Verification items for the finished model (mm, model axes). A direction names the side the tool comes from. Round coordinates to 2 decimals unless told otherwise and drop trailing zeros. Loops run counter-clockwise (first coordinate to the right, second up) from the corner with the lowest first, then second, coordinate; pieces in that order, holes last. Notation, with made-up numbers: M 14,43 L 57,43 A25 ccw 57,73 Z; hole C 63,53 d10. An arc over 180 degrees is marked long. One line per item, written item: value.
from build123d import *

# Parameters (mm, degrees)
SKETCH1_R               = 8
BOSS_EXTRUDE1_DEPTH     = 16
SKETCH2_R               = 6.5
CUT_EXTRUDE1_DEPTH      = 5
SKETCH3_R               = 5
CUT_EXTRUDE2_DEPTH      = 12
SKETCH4_R               = 1.25
CUT_EXTRUDE3_DEPTH      = 9
CUT_EXTRUDE3_DEPTH_BACK = 9
CUT_EXTRUDE5_START      = -10.5
SKETCH5_R               = 8
SKETCH5_R_2             = 7.25
CUT_EXTRUDE5_DEPTH      = 0.75
CUT_EXTRUDE6_START      = -12
SKETCH5_3_R             = 8
SKETCH5_3_R_2           = 7.25
CUT_EXTRUDE6_DEPTH      = 0.75


with BuildPart() as part:
    # Sketch1 → Boss-Extrude1 (new body)
    with BuildSketch(Plane(origin=(0, 0, 0), x_dir=(1, 0, 0), z_dir=(0, 1, 0))):
        Circle(SKETCH1_R)
    extrude(amount=BOSS_EXTRUDE1_DEPTH)

    # Sketch2 → Cut-Extrude1 (cut)
    with BuildSketch(Plane.XZ):
        Circle(SKETCH2_R)
    extrude(amount=-CUT_EXTRUDE1_DEPTH, mode=Mode.SUBTRACT)

    # Sketch3 → Cut-Extrude2 (cut)
    with BuildSketch(Plane.XZ):
        Circle(SKETCH3_R)
    extrude(amount=-CUT_EXTRUDE2_DEPTH, mode=Mode.SUBTRACT)

    # Sketch4 → Cut-Extrude3 (cut, two sides)
    with BuildSketch(Plane.XY) as cut_extrude3_sk:
        with Locations((0, 8)):
            Circle(SKETCH4_R)
    extrude(amount=CUT_EXTRUDE3_DEPTH, mode=Mode.SUBTRACT)
    extrude(cut_extrude3_sk.sketch, amount=-CUT_EXTRUDE3_DEPTH_BACK, mode=Mode.SUBTRACT)

    # Sketch5 → Cut-Extrude5 (cut)
    with BuildSketch(Plane.XZ.offset(CUT_EXTRUDE5_START)):
        Circle(SKETCH5_R)
        Circle(SKETCH5_R_2, mode=Mode.SUBTRACT)
    extrude(amount=-CUT_EXTRUDE5_DEPTH, mode=Mode.SUBTRACT)

    # Sketch5<3> → Cut-Extrude6 (cut)
    with BuildSketch(Plane.XZ.offset(CUT_EXTRUDE6_START)):
        Circle(SKETCH5_3_R)
        Circle(SKETCH5_3_R_2, mode=Mode.SUBTRACT)
    extrude(amount=-CUT_EXTRUDE6_DEPTH, mode=Mode.SUBTRACT)


solid = part.part
(1) Sectioned sample at A-A on y = 8. Enter the section's corners in (x, z), and give its area (3 significant figures).
Completed:
outline: M -1.25,-7.9 L -1.25,-4.84 A5 cw -1.25,4.84 L -1.25,7.9 A8 ccw Z; M 1.25,-7.9 A8 ccw 1.25,7.9 L 1.25,4.84 A5 cw 1.25,-4.84 Z
area: 107 mm^2
(2) Sectioned sample at C-C on x = 0. Count the separate pieces of the cut face and the enclosed holes in it, and give its area (3 significant figures).
Completed:
separate pieces: 3
enclosed holes: 0
area: 104 mm^2
(3) Thickness scan on L1, parallel to Z at x = 0, y = 2; L2, parallel to Y at x = 5.25, z = -6; L3, parallel to Y at x = 0, z = -7.1. Record the ranges inside material, lowest first. Write a range as from..to.
Completed:
L1: z = -8..-6.5, 6.5..8
L2: y = 0..10.5, 11.25..12, 12.75..16
L3: y = 0..6.75, 9.25..16
(4) Sectioned sample at B-B on z = 0. Enter the section's corners in (x, y), and give its area (3 significant figures).
Completed:
outline: M -8,0 L -6.5,0 L -6.5,5 L -5,5 L -5,12 L 5,12 L 5,5 L 6.5,5 L 6.5,0 L 8,0 L 8,10.5 L 7.25,10.5 L 7.25,11.25 L 8,11.25 L 8,12 L 7.25,12 L 7.25,12.75 L 8,12.75 L 8,16 L -8,16 L -8,12.75 L -7.25,12.75 L -7.25,12 L -8,12 L -8,11.25 L -7.25,11.25 L -7.25,10.5 L -8,10.5 Z
area: 119 mm^2
(5) Mould release check, pull along Z, two halves, no side actions. Record for faces 1 (the face through (1.155, 7.521, -6.398)), 2 (the face through (-5.158, 2.465, -3.955)), 3 (the face through (0, 12, 0)), 4 (the face through (-1.73, 11.62, 7.81)): +Z half, -Z half, draft (parallel to the pull), parting line (faces both ways), or undercut.
Completed:
face 1: draft
face 2: undercut
face 3: undercut
face 4: parting line
(6) Tool access check on faces 5 (the face through (4.619, 8.451, -1.915)), 6 (the face through (-1.73, 14.35, 7.81)), 7 (the face through (3.35, 10.87, -6.43)). Record the directions out of +Z, -Z, +X, -X, +Y, -Y that give a thin tool (end or side, any length) a straight path to the whole face; none if there is none.
Completed:
face 5: -Y
face 6: +Y, -Y
face 7: none
(7) Depth check by flat-ended pin: pin 1 Ø4 at (y, z) = (12.5, 2.5) entering from +X; pin 2 Ø6 at (y, z) = (13.5, 6) entering from -X; pin 3 Ø1.5 at (x, y) = (-2, 5.5) entering from -Z. Enter the tip coordinate at first touch or a pass-through.
Completed:
pin 1: stops at x = 7.98
pin 2: stops at x = -7.42
pin 3: stops at z = -7.9
(8) Sectioned sample at D-D on z = -5.75. Enter the section's corners in (x, y), and give its area (3 significant figures).
Completed:
outline: M -5.56,0 L -3.03,0 L -3.03,5 L 3.03,5 L 3.03,0 L 5.56,0 L 5.56,10.5 L 4.42,10.5 L 4.42,11.25 L 5.56,11.25 L 5.56,12 L 4.42,12 L 4.42,12.75 L 5.56,12.75 L 5.56,16 L -5.56,16 L -5.56,12.75 L -4.42,12.75 L -4.42,12 L -5.56,12 L -5.56,11.25 L -4.42,11.25 L -4.42,10.5 L -5.56,10.5 Z; hole C 0,8 d2.5
area: 139 mm^2
